```python
from build123d import *

# Parameters (mm, degrees)
F0_R     = 3.175
F1_DEPTH = 3.048


with BuildPart() as f1:
    # F0 (on Front) → F1 (new body)
    with BuildSketch(Plane.XZ):
        with BuildLine():
            ThreePointArc((0.677344, -9.500886), (6.970557, -6.491299), (9.525, 0))
            ThreePointArc((9.525, 0), (-0.476848, 9.513056), (-9.477255, -0.9525))
            ThreePointArc((-9.477255, -0.9525), (-6.389564, -7.063929), (0, -9.525))
            Line((0, -9.525), (0.677344, -9.500886))
        make_face()
        Circle(F0_R, mode=Mode.SUBTRACT)
        with BuildLine():
            ThreePointArc((-9.477255, -0.9525), (-0.476848, 9.513056), (9.525, 0))
            ThreePointArc((9.525, 0), (6.970557, -6.491299), (0.677344, -9.500886))
            Line((0.677344, -9.500886), (44.732405, -7.932475))
            ThreePointArc((44.732405, -7.932475), (36.513756, -0.141225), (44.45, 7.9375))
            Line((44.45, 7.9375), (19.13814, 7.9375))
            ThreePointArc((19.13814, 7.9375), (13.245391, 10.550923), (11.22682, 16.673))
            Line((11.22682, 16.673), (15.565216, 60.379155))
            ThreePointArc((15.565216, 60.379155), (-0.775265, 47.643942), (-15.795426, 61.9125))
            Line((-15.795426, 61.9125), (-9.477255, -0.9525))
        make_face()
        with BuildLine():
            ThreePointArc((0, -9.525), (0.338886, -9.51897), (0.677344, -9.500886))
            Line((0.677344, -9.500886), (0, -9.525))
        make_face()
        with BuildLine():
            ThreePointArc((-15.776702, 65.263889), (-15.874752, 63.58869), (-15.795426, 61.9125))
            ThreePointArc((-15.795426, 61.9125), (-0.775265, 47.643942), (15.565216, 60.379155))
            Line((15.565216, 60.379155), (15.875, 63.5))
            ThreePointArc((15.875, 63.5), (15.850406, 64.383313), (15.776702, 65.263889))
            ThreePointArc((15.776702, 65.263889), (0, 79.375), (-15.776702, 65.263889))
        make_face()
        with Locations((0, 63.5)):
            Circle(F0_R, mode=Mode.SUBTRACT)
        with BuildLine():
            ThreePointArc((44.45, 7.9375), (36.513756, -0.141225), (44.732405, -7.932475))
            ThreePointArc((44.732405, -7.932475), (50.161633, -5.51191), (52.3875, 0))
            ThreePointArc((52.3875, 0), (50.06266, 5.61266), (44.45, 7.9375))
        make_face()
        with Locations((44.45, 0)):
            Circle(F0_R, mode=Mode.SUBTRACT)
        with BuildLine():
            Line((-9.466021, 121.708333), (-15.776702, 65.263889))
            ThreePointArc((-15.776702, 65.263889), (0, 79.375), (15.776702, 65.263889))
            Line((15.776702, 65.263889), (9.466021, 121.708333))
            ThreePointArc((9.466021, 121.708333), (9.510244, 121.179988), (9.525, 120.65))
            ThreePointArc((9.525, 120.65), (-0.529988, 111.139756), (-9.466021, 121.708333))
        make_face()
        with Locations((-3.175, 100.0252)):
            Circle(F0_R, mode=Mode.SUBTRACT)
        with BuildLine():
            Line((15.875, 63.5), (15.565216, 60.379155))
            ThreePointArc((15.565216, 60.379155), (15.797364, 61.931909), (15.875, 63.5))
        make_face()
        with BuildLine():
            ThreePointArc((9.466021, 121.708333), (0, 130.175), (-9.466021, 121.708333))
            ThreePointArc((-9.466021, 121.708333), (-0.529988, 111.139756), (9.525, 120.65))
            ThreePointArc((9.525, 120.65), (9.510244, 121.179988), (9.466021, 121.708333))
        make_face()
        with Locations((0, 120.65)):
            Circle(F0_R, mode=Mode.SUBTRACT)
    extrude(amount=F1_DEPTH)


solid = f1.part
```
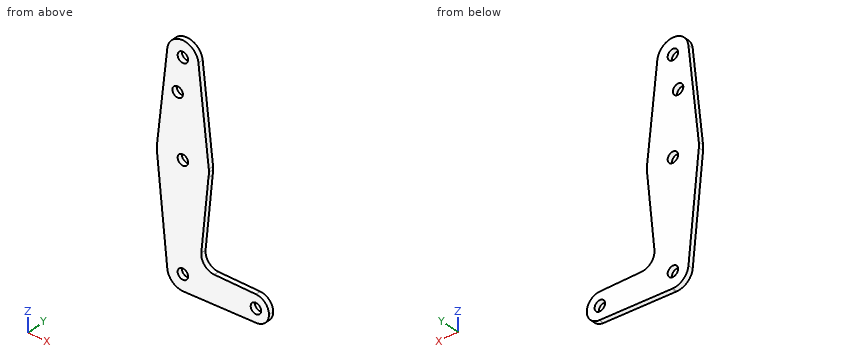
The model under review builds one solid part; all positions refer to its coordinate system, in mm. Round coordinates to 2 decimals unless told otherwise and drop trailing zeros. Loops run counter-clockwise (first coordinate to the right, second up) from the corner with the lowest first, then second, coordinate; pieces in that order, holes last. Notation, with made-up numbers: M -19.75,-24.75 L 29.25,-24.75 A36 ccw 29.25,14.25 Z; hole C -19.5,-19.5 d8. An arc over 180 degrees is marked long. Write item = value, one per line.
Item 1: Take a section at B-B on x = 27. Write out the cut boundary in (y, z).
Return value:
outline = M -3.05,-8.56 L 0,-8.56 L 0,7.94 L -3.05,7.94 Z
Item 2: Insertion check: P1, Ø1.5, axis at x = -2.5, y = -1, coming from the +Z side; P2, Ø1.5, axis at y = -1.5, z = 14, coming from the -X side; P3, Ø1, axis at x = -1.5, y = -1.5, coming from the -Z side. Each pin has a flat end and moves straight along its axis. Give the tip position at first contact, or say it passes through.
Return value:
P1 = 130.01
P2 = -11.06
P3 = -9.47
Item 3: Take a section at A-A on y = -1.65. State how many separate pieces and enclosed holes the cut face has, then the cut area to 3 significant figures.
Return value:
separate_pieces = 1
enclosed_holes = 5
area = 3,910 mm2
Item 4: For line 1 (Z direction, x = 2.5, y = -2.55); line 2 (X direction, y = -2.15, z = 0.5); line 3 (Z direction, x = 44.45, y = -1.9) (1 decimal), list the stretches that pass through material, from the lowest coordinate up. Write a range as [from, to].
Return value:
line_1 = [-9.44, -1.96], [1.96, 61.54], [65.46, 118.69], [122.61, 129.84]
line_2 = [-9.62, -3.14], [3.14, 41.31], [47.59, 52.37]
line_3 = [-7.9, -3.2], [3.2, 7.9]
Item 5: Take a section at C-C on z = 77. Write out the cut boundary in (x, y), then the cut area to 3 significant figures.
Return value:
outline = M -14.46,-3.05 L 14.46,-3.05 L 14.46,0 L -14.46,0 Z
area = 88.2 mm2
